CAD build for the part. Positions are in the model's coordinates, mm. Coordinates: 2 decimals unless noted, no trailing zeros. Loops run counter-clockwise (first coordinate to the right, second up) from the corner with the lowest first, then second, coordinate; pieces in that order, holes last. Notation, with made-up numbers: (-33, 22.25) - (9, 22.25) arc R26 cw to (9, 39.25) - close; hole circle Ø10 at (83, -20.75). An arc over 180 degrees is marked (long way). Put each result on its own line as item: value.
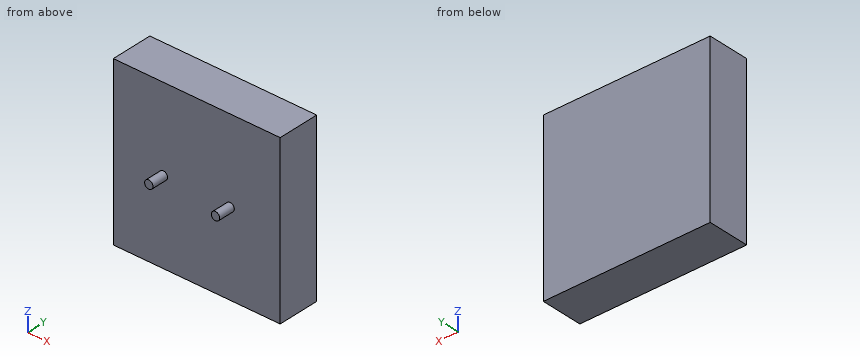
```python
from build123d import *

# Parameters (mm, degrees)
F0_W          = 10
F0_H          = 40
F1_DEPTH      = 20
F1_DEPTH_BACK = 20
F2_R          = 1
F3_DEPTH      = 4


with BuildPart() as f1:
    # F0 (on Right) → F1 (new body, two sides)
    with BuildSketch(Plane.YZ) as f1_sk:
        Rectangle(F0_W, F0_H)
    extrude(amount=F1_DEPTH)
    extrude(f1_sk.sketch, amount=-F1_DEPTH_BACK)

    # F2 (on face) → F3 (join)
    with BuildSketch(Plane.XZ.offset(5)):
        with Locations((-8, 0)):
            Circle(F2_R)
        with Locations((8, 0)):
            Circle(F2_R)
    extrude(amount=F3_DEPTH)


solid = f1.part
```
Q1. Wall check: L1, parallel to Y at x = -0.5, z = -16. Give the ranges that are in metal, low to high. Write a range as from..to.
Determined:
L1: -5..5
Q2. Slice it at C-C, the plane z = -14.5. Give the cut face in (x, y).
Determined:
outline: (-20, -5) - (20, -5) - (20, 5) - (-20, 5) - close
Q3. Slice it at D-D, the plane x = -12. Give the cut face in (y, z).
Determined:
outline: (-5, -20) - (5, -20) - (5, 20) - (-5, 20) - close
Q4. Slice it at B-B, the plane y = -7.25. Give the cut face in (x, z), then the cut area to 3 significant figures.
Determined:
outline: circle Ø2 at (-8, 0); circle Ø2 at (8, 0)
area: 6.28 mm2
Q5. Pin check, flat tip, straight feed: pin 1 Ø3 at (x, z) = (8.5, 4) entering from -Y. Stop position of the tip, or through.
Determined:
pin 1: y = -5
Q6. Slice it at A-A, the plane x = -8. Give the cut face in (y, z).
Determined:
outline: (-9, -1) - (-5, -1) - (-5, -20) - (5, -20) - (5, 20) - (-5, 20) - (-5, 1) - (-9, 1) - close
